Design review of the part built by this model. Coordinates are the model's own, in mm. Face numbers are marked on the shaded views. A direction names the side the tool comes from. Give positions to 0.01 mm unless a question says otherwise; leave off trailing zeros. Loops run counter-clockwise (first coordinate to the right, second up) from the corner with the lowest first, then second, coordinate; pieces in that order, holes last. Notation, with made-up numbers: (57, 67.5) -> (114, 67.5) arc R33 ccw to (114, 98.5) -> close; hole circle Ø7 at (18, 57). An arc over 180 degrees is marked (long way). Answer as CSV lines item,"result".
Autodesk Inventor part; units mm, degrees
ref_plane "YZ Plane" through (0, 0, 0) normal (1, 0, 0) x (0, 1, 0)
ref_plane "XZ Plane" through (0, 0, 0) normal (0, 1, 0) x (-1, 0, 0)
ref_plane "XY Plane" through (0, 0, 0) normal (0, 0, 1) x (1, 0, 0)
sketch "Sketch1" plane through (0, 0, 0) normal (1, 0, 0) x (0, 1, 0)
  line L0 (-47.625, 82.55) -> (-47.625, -82.55)
  line L1 (-47.625, -82.55) -> (47.625, -82.55)
  line L2 (47.625, -82.55) -> (47.625, 82.55)
  line L3 (47.625, 82.55) -> (-47.625, 82.55)
  line L4 (-47.625, 82.55) -> (47.625, -82.55) construction
  line L5 (-47.625, -82.55) -> (47.625, 82.55) construction
  point P0 (0, 0)
  dimension "d0" = 165.1
  dimension "d1" = 95.25
extrude "Extrusion1" add sketch "Sketch1" along normal mid plane 138.43
sketch "Sketch3" plane through (-69.215, 47.625, 82.55) normal (0, 1, 0) x (1, 0, 0)
  line L0 (0, 0) -> (138.43, 0)
  line L1 (138.43, 0) -> (138.43, 82.55)
  line L2 (138.43, 165.1) -> (138.43, 0)
  line L3 (1.27, 63.5) -> (137.16, 63.5)
  line L4 (137.16, 63.5) -> (137.16, 101.6)
  line L5 (137.16, 101.6) -> (1.27, 101.6)
  line L6 (1.27, 101.6) -> (1.27, 63.5)
  line L7 (1.27, 63.5) -> (137.16, 101.6) construction
  line L8 (137.16, 63.5) -> (1.27, 101.6) construction
  line L9 (2.54, 0) -> (133.35, 0)
  line L10 (133.35, 0) -> (133.35, 63.5)
  line L11 (133.35, 0) -> (133.35, 165.1)
  line L12 (133.35, 63.5) -> (2.54, 63.5)
  line L13 (2.54, 63.5) -> (2.54, 0)
  line L14 (2.54, 0) -> (133.35, 0)
  line L15 (133.35, 0) -> (133.35, 63.5)
  line L16 (2.54, 165.1) -> (2.54, 0)
  line L17 (2.54, 165.1) -> (2.54, 101.6)
  line L18 (2.54, 101.6) -> (133.35, 101.6)
  line L19 (133.35, 101.6) -> (133.35, 165.1)
  line L20 (133.35, 165.1) -> (2.54, 165.1)
  line L21 (2.54, 165.1) -> (2.54, 101.6)
  point P0 (69.215, 82.55)
  point P1 (2.54, 101.6)
  point P2 (133.35, 101.6)
  dimension "d12" = 38.1
  dimension "d13" = 63.5
extrude "Extrusion3" cut sketch "Sketch3" against normal blind 12962.89 contours L13 L3 L10 L0 | L16 L20 L11 L5
sketch "Sketch4" plane through (69.215, 0, 0) normal (1, 0, 0) x (0, 0, -1)
  point P0 (0, 0)
sketch "Sketch5" plane through (-66.675, 47.625, 19.05) normal (0, 0, 1) x (1, 0, 0)
  line L0 (135.89, -95.25) -> (135.89, 0)
  line L1 (135.89, -95.25) -> (133.35, -95.25)
  line L2 (135.89, -95.25) -> (130.81, -95.25)
  line L3 (130.81, 0) -> (0, 0)
  line L4 (0, 0) -> (0, -2.54)
  line L5 (0, 0) -> (0, -95.25)
  line L6 (0, -2.54) -> (133.35, -2.54)
  line L7 (133.35, -2.54) -> (133.35, -95.25)
  line L8 (133.35, -95.25) -> (0, -95.25)
  line L9 (0, -95.25) -> (0, -2.54)
  point P0 (66.675, -47.625)
  dimension "d16" = 2.54
  dimension "d17" = 2.54
extrude "Extrusion4" cut sketch "Sketch5" along normal mid plane 203.2
sketch "Sketch7" plane through (-69.215, 47.625, 82.55) normal (0, 1, 0) x (1, 0, 0)
  line L0 (133.35, 63.5) -> (133.35, 0)
  line L1 (135.89, 0) -> (138.43, 0)
  line L2 (133.35, 63.5) -> (135.89, 63.5)
  line L3 (135.89, 63.5) -> (135.89, 0)
  line L4 (135.89, 0) -> (133.35, 0)
  line L5 (133.35, 0) -> (133.35, 63.5)
  line L6 (133.35, 101.6) -> (2.54, 101.6)
  line L7 (135.89, 0) -> (135.89, 165.1)
  line L8 (133.35, 101.6) -> (135.89, 101.6)
  line L9 (135.89, 101.6) -> (135.89, 165.1)
  line L10 (135.89, 165.1) -> (133.35, 165.1)
  line L11 (133.35, 165.1) -> (133.35, 101.6)
  point P0 (69.215, 82.55)
extrude "Extrusion5" cut sketch "Sketch7" against normal blind 25.4
sketch "Sketch8" plane through (-69.215, 0, 0) normal (-1, 0, 0) x (0, 0, 1)
  line L0 (-19.05, 45.085) -> (19.05, 45.085)
  line L1 (-19.05, 45.085) -> (19.05, 45.085)
  line L2 (-19.05, 45.085) -> (-25.4, 45.085)
  line L3 (-25.4, 45.085) -> (-76.2, 45.085)
  line L4 (-25.4, 45.085) -> (-31.75, 45.085)
  line L5 (-82.55, -47.625) -> (82.55, -47.625)
  line L6 (-31.75, 45.085) -> (-31.75, -47.625)
  line L7 (-31.75, -47.625) -> (-69.85, -47.625)
  line L8 (-69.85, -47.625) -> (-69.85, 45.085)
  line L9 (-69.85, 45.085) -> (-31.75, 45.085)
  line L10 (19.05, 45.085) -> (31.75, 45.085)
  line L11 (31.75, 45.085) -> (31.75, -47.625)
  line L12 (31.75, -47.625) -> (69.85, -47.625)
  line L13 (69.85, -47.625) -> (69.85, 45.085)
  line L14 (69.85, 45.085) -> (31.75, 45.085)
  point P0 (0, 0)
  point P1 (-69.85, 45.085)
  dimension "d22" = 6.35
  dimension "d23" = 50.8
  dimension "d24" = 6.35
  dimension "d25" = 38.1
  dimension "d26" = 12.7
  dimension "d27" = 38.1
extrude "Extrusion6" cut sketch "Sketch8" against normal blind 25.4 contours L14 L13 L5 L11 | L6 L5 L8 L3
sketch "Sketch9" plane through (-69.215, 47.625, 82.55) normal (0, 1, 0) x (1, 0, 0)
  line L0 (2.54, 101.6) -> (2.54, 165.1)
  line L1 (2.54, 165.1) -> (2.54, 158.75)
  line L2 (2.54, 158.75) -> (135.89, 158.75)
  line L3 (135.89, 158.75) -> (135.89, 165.1)
  line L4 (135.89, 165.1) -> (2.54, 165.1)
  line L5 (2.54, 0) -> (2.54, 63.5)
  line L6 (2.54, 0) -> (2.54, 6.35)
  line L7 (2.54, 6.35) -> (135.89, 6.35)
  line L8 (135.89, 6.35) -> (135.89, 0)
  line L9 (135.89, 0) -> (2.54, 0)
  point P0 (69.215, 82.55)
  dimension "d30" = 6.35
  dimension "d31" = 6.35
extrude "Extrusion7" add sketch "Sketch9" against normal blind 2.54
sketch "Sketch10" plane through (-69.215, 0, 0) normal (-1, 0, 0) x (0, 0, 1)
  line L0 (-69.85, 45.085) -> (-69.85, -47.625)
  line L1 (-69.85, -47.625) -> (-69.85, 41.275)
  line L2 (-69.85, 41.275) -> (69.85, 41.275)
  line L3 (69.85, -47.625) -> (69.85, 45.085)
  line L4 (-69.85, 45.085) -> (-31.75, 45.085)
  line L5 (-69.85, 41.275) -> (-69.85, 45.085)
  line L6 (-69.85, 45.085) -> (-31.75, 45.085)
  line L7 (-31.75, 45.085) -> (-31.75, 41.275)
  line L8 (-31.75, 41.275) -> (-69.85, 41.275)
  line L9 (31.75, 45.085) -> (31.75, -47.625)
  line L10 (69.85, 45.085) -> (31.75, 45.085)
  line L11 (31.75, 41.275) -> (69.85, 41.275)
  line L12 (69.85, 41.275) -> (69.85, 45.085)
  line L13 (69.85, 45.085) -> (31.75, 45.085)
  line L14 (31.75, 45.085) -> (31.75, 41.275)
  point P0 (0, 0)
  dimension "d34" = 88.9
extrude "Extrusion8" add sketch "Sketch10" against normal blind 2.54
sketch "Sketch11" plane through (-69.215, 47.625, 82.55) normal (0, 1, 0) x (1, 0, 0)
  line L0 (0, 165.1) -> (0, 152.4)
  line L1 (135.89, 101.6) -> (2.54, 101.6)
  line L2 (0, 158.75) -> (12.7, 158.75)
  line L3 (12.7, 158.75) -> (12.7, 101.6)
  line L4 (12.7, 101.6) -> (0, 101.6)
  line L5 (0, 101.6) -> (0, 158.75)
  line L6 (2.54, 63.5) -> (135.89, 63.5)
  line L7 (0, 6.35) -> (12.7, 6.35)
  line L8 (12.7, 6.35) -> (12.7, 63.5)
  line L9 (12.7, 63.5) -> (0, 63.5)
  line L10 (0, 63.5) -> (0, 6.35)
  line L11 (138.6414, 6.35) -> (125.9414, 6.35)
  line L12 (125.9414, 6.35) -> (125.9414, 63.5)
  line L13 (125.9414, 63.5) -> (138.6414, 63.5)
  line L14 (138.6414, 63.5) -> (138.6414, 6.35)
  line L15 (125.9414, 101.6) -> (138.6414, 101.6)
  line L16 (138.6414, 101.6) -> (138.6414, 158.75)
  line L17 (138.6414, 158.75) -> (125.9414, 158.75)
  line L18 (125.9414, 158.75) -> (125.9414, 101.6)
  point P0 (69.215, 82.55)
  dimension "d37" = 12.7
  dimension "d38" = 12.7
  dimension "d39" = 12.7
extrude "Extrusion9" add sketch "Sketch11" against normal blind 2.54
sketch "Sketch12" plane through (-69.215, 47.625, -82.55) normal (0, 1, 0) x (1, 0, 0)
  line L0 (138.43, 0) -> (138.43, -6.35)
  line L1 (138.43, -6.35) -> (125.73, -6.35)
  line L2 (125.9414, -6.35) -> (12.7, -6.35)
  line L3 (138.43, -158.75) -> (138.43, -165.1)
  line L4 (138.43, -6.35) -> (138.43, -165.1)
  line L5 (138.43, -165.1) -> (125.73, -165.1)
  line L6 (125.73, -165.1) -> (125.73, -6.35)
  line L7 (125.73, -6.35) -> (138.43, -6.35)
  point P0 (69.215, -82.55)
  dimension "d42" = 12.7
  dimension "d43" = 12.7
extrude "Extrusion10" add sketch "Sketch12" against normal blind 2.54
sketch "Sketch13" plane through (-69.215, 47.625, -82.55) normal (0, 1, 0) x (1, 0, 0)
  line L0 (125.73, -63.5) -> (125.73, -6.35)
  line L1 (12.7, -6.35) -> (125.73, -6.35)
  line L2 (125.73, -6.35) -> (12.7, -6.35)
  line L3 (12.7, -6.35) -> (12.7, 0)
  line L4 (12.7, 0) -> (125.73, 0)
  line L5 (125.73, 0) -> (125.73, -6.35)
  line L6 (125.73, -158.75) -> (125.73, -101.6)
  line L7 (12.7, -101.6) -> (12.7, -158.75)
  line L8 (125.73, -158.75) -> (12.7, -158.75)
  line L9 (12.7, -158.75) -> (12.7, -165.1)
  line L10 (12.7, -165.1) -> (125.73, -165.1)
  line L11 (125.73, -165.1) -> (125.73, -158.75)
  point P0 (69.215, -82.55)
extrude "Extrusion11" cut sketch "Sketch13" against normal blind 2.54
sketch "Sketch14" plane through (-69.215, 0, 0) normal (-1, 0, 0) x (0, 0, 1)
  circle A0 centre (0, -5.2326) radius 1.7859
  circle A1 centre (9.779, -15.0116) radius 1.7859
  circle A2 centre (-9.779, -15.0116) radius 1.7859
  circle A3 centre (0, -24.7906) radius 1.7859
  line L0 (82.55, 47.625) -> (-82.55, 47.625)
  circle A4 centre (0, 12.446) radius 1.7859
  circle A5 centre (9.779, 22.225) radius 1.7859
  circle A6 centre (-9.779, 22.225) radius 1.7859
  circle A7 centre (0, 32.004) radius 1.7859
  point P0 (0, 0)
  dimension "d49" = 3.5719
  dimension "d50" = 3.5719
  dimension "d51" = 3.5719
  dimension "d52" = 3.5719
  dimension "d71" = 3.5719
  dimension "d72" = 3.5719
  dimension "d73" = 3.5719
  dimension "d74" = 3.5719
extrude "Extrusion12" cut sketch "Sketch14" against normal blind 2.54
sketch "Sketch15" plane through (-69.215, 47.625, 82.55) normal (0, 1, 0) x (1, 0, 0)
  line L0 (138.43, 158.75) -> (138.6414, 158.75)
  line L1 (138.43, 158.75) -> (138.6414, 158.75)
  line L2 (138.6414, 158.75) -> (138.6414, -0.8057)
  line L3 (138.6414, -0.8057) -> (138.43, -0.8057)
  line L4 (138.43, -0.8057) -> (138.43, 158.75)
  point P0 (69.215, 82.55)
extrude "Extrusion13" cut sketch "Sketch15" against normal blind 152.4
sketch "Sketch16" plane through (69.215, 47.625, 82.55) normal (0, 1, 0) x (1, 0, 0)
  line L0 (-125.73, 101.6) -> (-125.73, 165.1)
  line L1 (-125.73, 165.1) -> (-81.28, 165.1)
  line L2 (-81.28, 165.1) -> (-81.28, 0)
  line L3 (-81.28, 0) -> (-125.73, 0)
  line L4 (-125.73, 0) -> (-125.73, 165.1)
  point P0 (-69.215, 82.55)
  dimension "d57" = 44.45
extrude "Extrusion14" add sketch "Sketch16" against normal blind 2.54
sketch "Sketch17" plane through (69.215, -47.625, -82.55) normal (0, 0, -1) x (-1, 0, 0)
  line L0 (2.54, 0) -> (0, 0)
  line L1 (0, 0) -> (1.27, 0)
  line L2 (1.27, 0) -> (3.81, 0)
  line L3 (3.81, 0) -> (3.81, 95.25)
  line L4 (3.81, 95.25) -> (1.27, 95.25)
  line L5 (1.27, 95.25) -> (1.27, 0)
  point P0 (69.215, 47.625)
  dimension "d60" = 1.27
  dimension "d61" = 2.54
extrude "Extrusion15" add sketch "Sketch17" against normal blind 165.1
sketch "Sketch18" plane through (69.215, -47.625, -82.55) normal (0, 0, -1) x (-1, 0, 0)
  line L0 (0, 0) -> (3.81, 0)
  line L1 (0, 0) -> (1.27, 0)
  line L2 (1.27, 0) -> (1.27, 95.25)
  line L3 (1.27, 95.25) -> (0, 95.25)
  line L4 (0, 95.25) -> (0, 0)
  point P0 (69.215, 47.625)
  dimension "d64" = 1.27
extrude "Extrusion16" cut sketch "Sketch18" against normal blind 165.1
sketch "Sketch19" plane through (56.515, 47.625, -82.55) normal (-1, 0, 0) x (0, 0, 1)
  line L0 (0, -2.54) -> (0, 0)
  line L1 (101.6, 0) -> (165.1, 0)
  line L2 (0, 0) -> (165.1, 0)
  line L3 (165.1, 0) -> (165.1, -2.5502)
  line L4 (165.1, -2.5502) -> (0, -2.5502)
  line L5 (0, -2.5502) -> (0, 0)
  point P0 (82.55, -47.625)
extrude "Extrusion17" add sketch "Sketch19" along normal blind 1.27
equation "\"d49\" = d51"
properties part number "intakeCover"
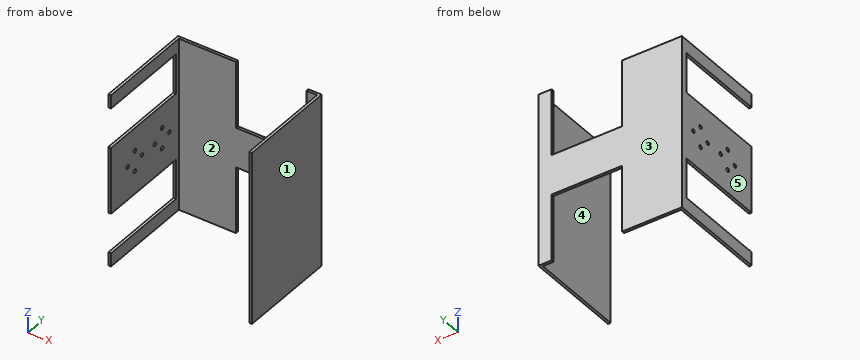
Q1. Clearance check with flat-ended pins moving along their axes: pin 1 Ø1 at (x, z) = (56, -3.5) entering from -Y; pin 2 Ø2 at (y, z) = (22.225, 9.779) entering from -X (3 decimals). State where each tip first meets the part, or that it passes through.
Filled sheet:
pin 1,"stops at y = 45.07"
pin 2,"stops at x = 65.405"
Q2. To check wall thickness, follow probe 1 along Y at (x, z) = (-68.6, 0) (1 decimal); probe 2 along X at (y, z) = (31, 8) (3 decimals); probe 3 along X at (y, z) = (-39, 60) (3 decimals). State the ranges of each line that lie inside material, in increasing order. Write a range as from..to.
Filled sheet:
probe 1,"y = -47.6..-26.6, -23..-7, -3.4..10.7, 14.2..30.2, 33.8..47.6"
probe 2,"x = -69.215..-66.675, 65.405..67.945"
probe 3,"x = 65.405..67.945"
Q3. We need section C-C, the plane z = 5.5. State the section outline as (x, y) points (3 decimals), and give its area (3 significant figures).
Filled sheet:
outline,"(-69.215, -47.625) -> (-66.675, -47.625) -> (-66.675, 45.085) -> (55.245, 45.085) -> (55.245, 45.075) -> (56.515, 45.075) -> (56.515, 45.085) -> (65.405, 45.085) -> (65.405, -47.625) -> (67.945, -47.625) -> (67.945, 47.625) -> (-69.215, 47.625) -> close"
area,"819 mm^2"
Q4. We need section D-D, the plane x = 31.5. State the section outline as (y, z) points (3 decimals), and give its area (3 significant figures).
Filled sheet:
outline,"(45.085, -19.05) -> (47.625, -19.05) -> (47.625, 19.05) -> (45.085, 19.05) -> close"
area,"96.8 mm^2"
Q5. For the marked faces 1 and 2, list the 3-axis set-ups (+Z, -Z, +X, -X, +Y, -Y) from which the entire face can be reached by the end or side of a thin tool; tool diameter is ignored.
Filled sheet:
face 1,"+Z, -Z, +X, +Y, -Y"
face 2,"+Z, -Z, -Y"
Q6. The part is to be moulded in two halves that separate along X. For the marked faces 3, 4 and 5, say which applies: pulls with the +X half, pulls with the -X half, needs draft (parallel to the pull), parting line crosses it, or undercut.
Filled sheet:
face 3,"needs draft"
face 4,"undercut"
face 5,"pulls with the -X half"
Q7. We need section A-A, the plane y = -20.5. State the section outline as (x, z) points (3 decimals).
Filled sheet:
outline,"(-69.215, -82.55) -> (-66.675, -82.55) -> (-66.675, -69.85) -> (-69.215, -69.85) -> close; (-69.215, -31.75) -> (-66.675, -31.75) -> (-66.675, 31.75) -> (-69.215, 31.75) -> close; (-69.215, 69.85) -> (-66.675, 69.85) -> (-66.675, 82.55) -> (-69.215, 82.55) -> close; (65.405, -82.55) -> (67.945, -82.55) -> (67.945, 82.55) -> (65.405, 82.55) -> close"
Q8. We need section B-B, the plane z = 72.5. State the section outline as (x, y) points (3 decimals), and give its area (3 significant figures).
Filled sheet:
outline,"(-69.215, -47.625) -> (-66.675, -47.625) -> (-66.675, 45.085) -> (-12.065, 45.085) -> (-12.065, 47.625) -> (-69.215, 47.625) -> close; (55.245, 45.075) -> (56.515, 45.075) -> (56.515, 45.085) -> (65.405, 45.085) -> (65.405, -47.625) -> (67.945, -47.625) -> (67.945, 47.625) -> (55.245, 47.625) -> close"
area,"648 mm^2"
